Autodesk Inventor part; units mm, degrees
ref_plane "YZ Plane" through (0, 0, 0) normal (1, 0, 0) x (0, 1, 0)
ref_plane "XZ Plane" through (0, 0, 0) normal (0, 1, 0) x (-1, 0, 0)
ref_plane "XY Plane" through (0, 0, 0) normal (0, 0, 1) x (1, 0, 0)
sketch "Schizzo1" plane through (0, 0, 0) normal (0, 0, 1) x (1, 0, 0)
  line L0 (0, 0) -> (90, 0)
  line L1 (90, 0) -> (90, -121)
  line L2 (90, -121) -> (0, -121)
  line L3 (0, -121) -> (0, 0)
  dimension "d0" = 90
  dimension "d1" = 121
extrude "Estrusione1" add sketch "Schizzo1" along normal blind 1
sketch "Schizzo2" plane through (0, 0, 0) normal (0, 0, -1) x (-1, 0, 0)
  line L0 (-90, 0) -> (-90, -32)
  line L1 (-90, -121) -> (-90, 0)
  line L2 (-81, -32) -> (-66, -32)
  line L3 (-66, -32) -> (-66, -50)
  line L4 (-66, -50) -> (-81, -50)
  line L5 (-81, -50) -> (-81, -32)
  line L6 (-90, 0) -> (-90, -40)
  line L7 (-51, -40) -> (-29, -40)
  line L8 (-29, -40) -> (-29, -70)
  line L9 (-29, -70) -> (-51, -70)
  line L10 (-51, -70) -> (-51, -40)
  dimension "d10" = 22
  dimension "d11" = 30
extrude "Estrusione2" add sketch "Schizzo2" along normal blind 20
sketch "Schizzo3" plane through (0, 0, 1) normal (0, 0, 1) x (1, 0, 0)
  line L0 (90, -121) -> (90, 0)
  line L1 (90, 0) -> (90, -19)
  line L2 (87, -19) -> (7, -19)
  line L3 (7, -19) -> (7, -54)
  line L4 (7, -54) -> (87, -54)
  line L5 (87, -54) -> (87, -19)
  line L6 (90, -121) -> (90, -100)
  line L7 (87, -100) -> (3, -100)
  line L8 (3, -100) -> (3, -65)
  line L9 (3, -65) -> (87, -65)
  line L10 (87, -65) -> (87, -100)
  dimension "d16" = 80
  dimension "d17" = 35
  dimension "d19" = 84
  dimension "d20" = 35
extrude "Estrusione3" add sketch "Schizzo3" along normal blind 30
sketch "Schizzo4" plane through (0, 0, 1) normal (0, 0, 1) x (1, 0, 0)
  line L0 (90, -121) -> (90, 0)
  line L1 (90, 0) -> (90, -6)
  circle A0 centre (86, -6) radius 2
  circle A1 centre (4, -6) radius 2
  circle A2 centre (86, -106) radius 2
  circle A3 centre (4, -106) radius 2
  dimension "d28" = 4
  dimension "d32" = 4
  dimension "d33" = 4
extrude "Estrusione4" cut sketch "Schizzo4" against normal up to surface (1 mm away)
properties part number "pcb" material "Plastica ABS"
The listing builds one solid part. Answer for the finished solid, in the listing's coordinates (mm). A direction names the side the tool comes from. Round coordinates to 2 decimals unless told otherwise and drop trailing zeros. Write each loop counter-clockwise with the first axis right and the second up, starting at its lowest first coordinate (ties: lowest second). Pieces come first, ordered by that corner, then holes. Notation, with made-up numbers: (51.5, -23.5) -> (100.5, -23.5) arc R7 ccw to (100.5, -11.5) -> close; hole circle Ø6 at (6, 36). An arc over 180 degrees is marked (long way). Answer as a JSON object with one key per item and string values. Group by question number.
Q1. Section D-D (y = -41.5) is taken. Write down the section's boundary in (x, z).
Q2. Section A-A (z = -6) is taken. Write down the section's boundary in (x, y).
Q3. Determine the mould class of faces 4 (the face through (3.74, -104.017, 0.507)), 5 (the face through (46, -100, 16)), 6 (the face through (3, -83, 16)) for opening direction Y: pulls with the +Y half, pulls with the -Y half, needs draft (parallel to the pull), parting line crosses it, or undercut.
Q4. Each of these flat-tipped pins is pushed along its axis until it touches: pin 1 Ø10 at (y, z) = (-52.5, -6) entering from +X; pin 2 Ø24 at (x, z) = (59, 12.5) entering from +Y; pin 3 Ø9 at (x, z) = (59.5, 23.5) entering from -Y; pin 4 Ø3 at (x, z) = (32.5, 12.5) entering from +Y. Where does it stop, or does it pass through?
Q5. Section C-C (x = 21) is taken. Write down the section's boundary in (y, z).
Q6. Which of the six approach directions +Z, -Z, +X, -X, +Y, -Y give full straight-line access (tool end or side, diameter ignored) to faces 1 (the face through (81, -41, -10)), 2 (the face through (73, -50, -10)), 3 (the face through (44, -65, 16))?
Q7. Straight lines are drawn through the part: line 1 along Y through (x, z) = (86, 0.7); line 2 along Y through (x, z) = (68, 21); line 3 along Y through (x, z) = (75, -17.5). For each, find the intervals that lie inside material, in ascending order.
Q8. Section B-B (y = -106) is taken. Write down the section's boundary in (x, z), plus the area to 3 significant figures.
Check values:
{
 "1": {"outline": "(0, 0) -> (29, 0) -> (29, -20) -> (51, -20) -> (51, 0) -> (66, 0) -> (66, -20) -> (81, -20) -> (81, 0) -> (90, 0) -> (90, 1) -> (87, 1) -> (87, 31) -> (7, 31) -> (7, 1) -> (0, 1) -> close"},
 "2": {"outline": "(29, -70) -> (51, -70) -> (51, -40) -> (29, -40) -> close; (66, -50) -> (81, -50) -> (81, -32) -> (66, -32) -> close"},
 "3": {"face 4": "undercut", "face 5": "pulls with the -Y half", "face 6": "needs draft"},
 "4": {"pin 1": "x = 81", "pin 2": "y = 0", "pin 3": "y = -100", "pin 4": "y = -19"},
 "5": {"outline": "(-121, 0) -> (0, 0) -> (0, 1) -> (-19, 1) -> (-19, 31) -> (-54, 31) -> (-54, 1) -> (-65, 1) -> (-65, 31) -> (-100, 31) -> (-100, 1) -> (-121, 1) -> close"},
 "6": {"face 1": "-Z, +X, +Y, -Y", "face 2": "-Z, +X, -Y", "face 3": "+Z, +X, -X"},
 "7": {"line 1": "-121 to -108, -104 to -8, -4 to 0", "line 2": "-100 to -65, -54 to -19", "line 3": "-50 to -32"},
 "8": {"outline": "(0, 0) -> (2, 0) -> (2, 1) -> (0, 1) -> close; (6, 0) -> (84, 0) -> (84, 1) -> (6, 1) -> close; (88, 0) -> (90, 0) -> (90, 1) -> (88, 1) -> close", "area": "82.0 mm^2"}
}
